Could you check a few things on this model? Use its own coordinates, in mm. A direction names the side the tool comes from. Give positions to 0.01 mm unless a question says otherwise; leave off trailing zeros. Write each loop counter-clockwise with the first axis right and the second up, starting at its lowest first coordinate (ties: lowest second). Pieces come first, ordered by that corner, then holes. Notation, with made-up numbers: M 23,21 L 75,21 A25 ccw 75,45 Z; hole C 60,-21.75 d8. An arc over 180 degrees is marked long. Write each question's results on one line, items separated by ' | '. Start each with the question number.
from build123d import *
from build123d.topology import SkipClean

# Parameters (mm, degrees)
SKETCH1_W               = 22
SKETCH1_H               = 12
BOSS_EXTRUDE1_DEPTH     = 6
FILLET1_R               = 0.2
SKETCH2_W               = 20.5
SKETCH2_H               = 10
CUT_EXTRUDE1_DEPTH      = 5
SKETCH3_R               = 1
SKETCH3_R_2             = 0.5
BOSS_EXTRUDE2_DEPTH     = 1
SKETCH7_R               = 1
SKETCH7_R_2             = 0.5
BOSS_EXTRUDE3_DEPTH     = 1
SKETCH8_R               = 0.5
CUT_EXTRUDE4_DEPTH      = 14.892443989
FILLET2_R               = 0.2
MIRROR5_COPY_1_SKETCH_R = 0.5
MIRROR5_COPY_1_DEPTH    = 14.892443989
SKETCH9_R               = 0.9
CUT_EXTRUDE12_DEPTH     = 1
MIRROR7_COPY_1_SKETCH_R = 0.9
MIRROR7_COPY_1_DEPTH    = 1


with BuildPart() as part:
    # Sketch1 → Boss-Extrude1 (new body)
    with BuildSketch(Plane(origin=(0, 0, 0), x_dir=(1, 0, 0), z_dir=(0, 1, 0))):
        Rectangle(SKETCH1_W, SKETCH1_H)
    extrude(amount=BOSS_EXTRUDE1_DEPTH)

    # Fillet1
    fillet1_edges = [part.edges().sort_by_distance(p)[0] for p in [
        (11, 3, 6),
        (-11, 3, 6),
        (-11, 3, -6),
        (11, 3, -6),
    ]]
    fillet(fillet1_edges, radius=FILLET1_R)

    # Sketch2 → Cut-Extrude1 (cut)
    with BuildSketch(Plane(origin=(0, 6, 0), x_dir=(1, 0, 0), z_dir=(0, 1, 0))):
        with Locations((-0.25, 0)):
            Rectangle(SKETCH2_W, SKETCH2_H)
    extrude(amount=-CUT_EXTRUDE1_DEPTH, mode=Mode.SUBTRACT)

    # Sketch3 → Boss-Extrude2 (add)
    with BuildSketch(Plane(origin=(0, 1, 0), x_dir=(1, 0, 0), z_dir=(0, 1, 0))):
        with Locations((10, 4.5)):
            Circle(SKETCH3_R)
        with Locations((10, 4.5)):
            Circle(SKETCH3_R_2, mode=Mode.SUBTRACT)
    boss_extrude2 = extrude(amount=BOSS_EXTRUDE2_DEPTH)

    # Mirror1: Boss-Extrude2 across plane
    add(boss_extrude2.mirror(Plane.XY))

    # Sketch7 → Boss-Extrude3 (add)
    with BuildSketch(Plane(origin=(0, 1, 0), x_dir=(1, 0, 0), z_dir=(0, 1, 0))):
        with Locations((-10, 4.5)):
            Circle(SKETCH7_R)
        with Locations(Location((-10, 4.5, 0), (0, 0, 90))):
            Circle(SKETCH7_R_2, mode=Mode.SUBTRACT)
    boss_extrude3 = extrude(amount=BOSS_EXTRUDE3_DEPTH)

    # Mirror3: Boss-Extrude3 across plane
    add(boss_extrude3.mirror(Plane.XY))

    # Sketch8 → Cut-Extrude4 (cut, through all)
    with SkipClean():  # the faces are left unmerged after this step: merging them gives an invalid solid
        with BuildSketch(Plane(origin=(0, 6, 0), x_dir=(1, 0, 0), z_dir=(0, 1, 0))):
            with Locations(Location((10, 4.5, 0), (0, 0, 270))):
                Circle(SKETCH8_R)
        cut_extrude4 = extrude(amount=-CUT_EXTRUDE4_DEPTH, mode=Mode.SUBTRACT)

    # Mirror4: Cut-Extrude4 across plane
    with SkipClean():  # the faces are left unmerged after this step: merging them gives an invalid solid
        add(cut_extrude4.mirror(Plane.XY), mode=Mode.SUBTRACT)

    # Fillet2
    fillet2_edges = [part.edges().sort_by_distance(p)[0] for p in [
        (10, 4, -4),
        (10, 4, 4),
    ]]
    fillet(fillet2_edges, radius=FILLET2_R)

    # Mirror5: Cut-Extrude4 across plane
    with SkipClean():  # the faces are left unmerged after this step: merging them gives an invalid solid
        add(cut_extrude4.mirror(Plane(origin=(0, 0, 0), x_dir=(0, 0, 1), z_dir=(1, 0, 0))), mode=Mode.SUBTRACT)

    # Mirror5 copy 1 sketch → Mirror5 copy 1 (cut, through all)
    with SkipClean():  # the faces are left unmerged after this step: merging them gives an invalid solid
        with BuildSketch(Plane(origin=(0, 6, 0), x_dir=(-1, 0, 0), z_dir=(0, 1, 0))):
            with Locations(Location((10, 4.5, 0), (0, 0, 270))):
                Circle(MIRROR5_COPY_1_SKETCH_R)
        extrude(amount=-MIRROR5_COPY_1_DEPTH, mode=Mode.SUBTRACT)

    # Sketch9 → Cut-Extrude12 (cut)
    with SkipClean():  # the faces are left unmerged after this step: merging them gives an invalid solid
        with BuildSketch(Plane(origin=(0, 0, 0), x_dir=(-1, 0, 0), z_dir=(0, -1, 0))):
            with Locations(Location((-10, -4.5, 0), (0, 0, 90))):
                Circle(SKETCH9_R)
        cut_extrude12 = extrude(amount=-CUT_EXTRUDE12_DEPTH, mode=Mode.SUBTRACT)

    # Mirror6: Cut-Extrude12 across plane
    with SkipClean():  # the faces are left unmerged after this step: merging them gives an invalid solid
        add(cut_extrude12.mirror(Plane(origin=(0, 0, 0), x_dir=(0, 0, 1), z_dir=(1, 0, 0))), mode=Mode.SUBTRACT)

    # Mirror7: Cut-Extrude12 across plane
    add(cut_extrude12.mirror(Plane.XY), mode=Mode.SUBTRACT)

    # Mirror7 copy 1 sketch → Mirror7 copy 1 (cut)
    with SkipClean():  # the faces are left unmerged after this step: merging them gives an invalid solid
        with BuildSketch(Plane.XZ):
            with Locations(Location((-10, -4.5, 0), (0, 0, 90))):
                Circle(MIRROR7_COPY_1_SKETCH_R)
        extrude(amount=-MIRROR7_COPY_1_DEPTH, mode=Mode.SUBTRACT)


solid = part.part
Q1. If we mould it in two halves opening along Z, with no side actions, what happens to faces 1 (the face through (-10.61, 0.49, 5.16)), 2 (the face through (0, 3, -6)), 3 (the face through (0, 0, 0))? For each: pulls with the +Z half, pulls with the -Z half, needs draft (parallel to the pull), parting line crosses it, or undercut.
Q2. If we section it at C-C (z = 1.75): Please give me the cut outline in (x, y), plus the area to 3 significant figures.
Q3. If we section it at B-B (x = -5.5): Please give me the cut outline in (y, z), plus the area to 3 significant figures.
Q4. I'm going to push flat-ended pins straight in: P1, Ø1.6, axis at x = 10, z = 4.5, coming from the -Y side; P2, Ø2, axis at x = -10.5, z = -4, coming from the -Y side; P3, Ø5, axis at x = 6.5, z = -1, coming from the +Y side; P4, Ø0.9, axis at x = 9.5, z = 4, coming from the +Y side. Where does each tip first touch, or does it pass through?
Q5. For faces 4 (the face through (-9.4, 2, -4.1)), 5 (the face through (10.61, 0.49, -5.16)), 6 (the face through (-11, 3, 0)), which set-ups out of +Z, -Z, +X, -X, +Y, -Y let a thin tool reach every point of the face, with its end or its side?
Q6. Please list where these lines run through material, in increasing order: line 1 (X direction, y = 1.45, z = -4.5); line 2 (X direction, y = 1.7, z = 0.75); line 3 (Z direction, x = -2.5, y = 4.8). Write a range as [from, to].
Q7. If we section it at D-D (z = 4.25): Please give me the cut outline in (x, y), plus the area to 3 significant figures.
Q8. If we section it at A-A (y = 3.45): Please give me the cut outline in (x, z).
Determined:
1) face 1: undercut | face 2: pulls with the -Z half | face 3: needs draft
2) outline: M -11,0 L 11,0 L 11,6 L 10,6 L 10,1 L -10.5,1 L -10.5,6 L -11,6 Z | area: 29.5 mm²
3) outline: M 0,-6 L 6,-6 L 6,-5 L 1,-5 L 1,5 L 6,5 L 6,6 L 0,6 Z | area: 22.0 mm²
4) P1: stops at y = 1 | P2: stops at y = 0 | P3: stops at y = 1 | P4: stops at y = 2
5) face 4: +Y | face 5: -Y | face 6: +Z, -Z, -X, +Y, -Y
6) line 1: x = [-11, -10.5], [-9.5, -9], [9, 9.5], [10.5, 11] | line 2: x = [-11, -10.5], [10, 11] | line 3: z = [-6, -5], [5, 6]
7) outline: M -11,0 L -10.86,0 L -10.86,1 L -10.43,1 L -10.43,2 L -10.5,2 L -10.5,6 L -11,6 Z; M -9.57,1 L -9.14,1 L -9.14,0 L 9.14,0 L 9.14,1 L 9.57,1 L 9.57,2 L 9.03,2 L 9.03,1 L -9.03,1 L -9.03,2 L -9.57,2 Z; M 10.43,1 L 10.86,1 L 10.86,0 L 11,0 L 11,6 L 10.43,6 Z | area: 25.0 mm²
8) outline: M -11,-5.8 A0.2 ccw -10.8,-6 L 10.8,-6 A0.2 ccw 11,-5.8 L 11,5.8 A0.2 ccw 10.8,6 L -10.8,6 A0.2 ccw -11,5.8 Z; hole M -10.5,-5 L 10,-5 A0.5 ccw 10.14,-4.02 A0.2 cw 10,-3.83 L 10,3.83 A0.2 cw 10.14,4.02 A0.5 ccw 10,5 L -10.5,5 Z
